The model under review builds one solid part; all positions refer to its coordinate system, in mm. A direction names the side the tool comes from. Round coordinates to 2 decimals unless told otherwise and drop trailing zeros. Write each loop counter-clockwise with the first axis right and the second up, starting at its lowest first coordinate (ties: lowest second). Pieces come first, ordered by that corner, then holes. Notation, with made-up numbers: (12.5, -11.75) - (23.5, -11.75) arc R9 ccw to (23.5, 0.25) - close; hole circle Ø8 at (75, 12.5). An arc over 180 degrees is marked (long way). Return JSON: item names as keys, results as strings.
from build123d import *

# Parameters (mm, degrees)
CUT_EXTRUDE1_DEPTH = 2


with BuildPart() as part:
    # Sketch1 → Revolve1 (revolve)
    with BuildSketch(Plane.XY):
        with BuildLine():
            Line((-0.8, 0), (-0.8, 2))
            Line((-0.8, 2), (-0.222649731, 3))
            Line((-0.222649731, 3), (0, 3))
            Line((0, 3), (0, 1.44675))
            ThreePointArc((0, 1.44675), (0.029289322, 1.376039322), (0.1, 1.34675))
            Line((0.1, 1.34675), (0.9, 1.34675))
            Line((0.9, 1.34675), (1.4, 1.5))
            Line((1.4, 1.5), (9.6935, 1.5))
            Line((9.6935, 1.5), (10, 1.1935))
            Line((10, 1.1935), (10, 0))
            Line((10, 0), (-0.8, 0))
        make_face()
    revolve(axis=Axis((10, 0, 0), (-1, 0, 0)))

    # Sketch2 → Cut-Revolve1 (revolve, cut)
    with BuildSketch(Plane.XY):
        Polygon((-0.8, 0), (-0.8, 0.75), (1.2, 0.75), (1.633012702, 0), align=None)
    revolve(axis=Axis((1.633012702, 0, 0), (-1, 0, 0)), mode=Mode.SUBTRACT)

    # Sketch3 → Cut-Extrude1 (cut)
    with BuildSketch(Plane(origin=(-0.8, 0, 0), x_dir=(0, 0, -1), z_dir=(1, 0, 0))):
        Polygon((-0.75, -0.433012702), (0, -0.866025404), (0.75, -0.433012702), (0.75, 0.433012702), (0, 0.866025404), (-0.75, 0.433012702), align=None)
    extrude(amount=CUT_EXTRUDE1_DEPTH, mode=Mode.SUBTRACT)


solid = part.part
(1) For faces 1 (the cylindrical face through (5.6, -1.5, -0.07)), 2 (the flat face through (0, 0, 0.75)), list the 3-axis set-ups (+Z, -Z, +X, -X, +Y, -Y) from which the entire face can be reached by the end or side of a thin tool; tool diameter is ignored.
Filled in:
{"face 1": "+X", "face 2": "-X"}
(2) Clearance check with flat-ended pins moving along their axes: pin 1 Ø1.5 at (x, z) = (5, 0.5) entering from -Y; pin 2 Ø1 at (x, z) = (6, 1) entering from -Y; pin 3 Ø1 at (y, z) = (-2.5, -0.5) entering from -X. State where each tip first meets the part, or that it passes through.
Filled in:
{"pin 1": "stops at y = -1.5", "pin 2": "stops at y = -1.41", "pin 3": "stops at x = -0.77"}
(3) Mouldability with a two-part tool opening along X and no side actions: class faces 3 (the cylindrical face through (0.51, -1.07, 0.82)), 4 (the flat face through (-0.8, 0, 1)), 5 (the flat face through (0, 0, -0.75)), 6 (the flat face through (10, 0, 0)) as released by +X, released by -X, zero draft, split by the parting line, or undercut.
Filled in:
{"face 3": "undercut", "face 4": "released by -X", "face 5": "zero draft", "face 6": "released by +X"}
(4) Add section B-B (x = 5.75). Write out the cut boundary in (y, z).
Filled in:
{"outline": "circle Ø3 at (0, 0)"}
(5) Add section A-A (x = 0.75). Write out the cut boundary in (y, z).
Filled in:
{"outline": "circle Ø2.69 at (0, 0); hole (-0.87, 0) - (-0.43, -0.75) - (0.43, -0.75) - (0.87, 0) - (0.43, 0.75) - (-0.43, 0.75) - close"}
(6) Wall thickness on line 1 (X direction, y = 0.45, z = 1.75); line 2 (X direction, y = 2.65, z = -1.3); line 3 (Z direction, x = 2, y = -0.2): over which ranges is each line inside the solid? List them lowest first.
Filled in:
{"line 1": "x = -0.8 to 0", "line 2": "x = -0.25 to 0", "line 3": "z = -1.49 to 1.49"}
